For this review, take the finished solid that the model builds, in its own axes (mm). A direction names the side the tool comes from. Give positions to 0.01 mm unless a question says otherwise; leave off trailing zeros. Order: outer loops, then holes, each group sorted by start corner. A loop starts at its lowest first (then second) coordinate and runs counter-clockwise, first axis right, second up. Notation, with made-up numbers: M 83.5,60 L 113.5,60 A16 cw 113.5,81 Z; hole C 63,57.25 d2. An arc over 180 degrees is marked long. Use CSV: the item, a comma, the result in double quotes. Start each with the question number.
(1) Consider section D-D (z = 17). Write out the cut boundary in (x, y), and give its area (3 significant figures).
(2) Consider section B-B (z = 3.5). Write out the cut boundary in (x, y), and give its area (3 significant figures).
(3) Draft analysis for pull direction X (two halves, no side actions). For faces 6 (the face through (30, 2, -37)), 7 (the face through (17.5, 1, 18)), 8 (the face through (-30, 2, 37)), state which applies: pulls with the +X half, pulls with the -X half, needs draft (parallel to the pull), parting line crosses it, or undercut.
(4) Consider section A-A (x = 35). Write out the cut boundary in (y, z), and give its area (3 significant figures).
(5) Wall thickness on L1, parallel to Z at x = 38.5, y = 1.2; L2, parallel to Z at x = -2.5, y = 1.5; L3, parallel to Z at x = 31, y = 3.3: over which ranges is each line inside the solid? List them lowest first. Write a range as from..to.
(6) Consider section C-C (x = 11). Write out the cut boundary in (y, z).
(7) Clearance check with flat-ended pins moving along their axes: P1, Ø1, axis at y = 2, z = 27, coming from the +X side; P2, Ø2, axis at y = 1.5, z = -36, coming from the -X side; P3, Ø0.6, axis at x = 37, y = 2, coming from the -Z side. State where each tip first meets the part, or that it passes through.
(8) Tool access review of faces 1 (the face through (0, 1, 13)), 2 (the face through (37, 2, 13.5)), 3 (the face through (-36, 2, 22.5)), 4 (the face through (-37, 2, 20.5)), 5 (the face through (-35, 2, -22.5)): name each direction out of +Z, -Z, +X, -X, +Y, -Y from which nothing blocks a thin tool from reaching the whole face with its end or side.
```python
from build123d import *

# Parameters (mm, degrees)
SALIENTE_EXTRUIR1_DEPTH = 4
CROQUIS2_W              = 55
CROQUIS2_H              = 101
CORTAR_EXTRUIR1_DEPTH   = 2
CROQUIS4_W              = 7
CROQUIS4_H              = 2
CORTAR_EXTRUIR2_DEPTH   = 9
CROQUIS6_W              = 7
CROQUIS6_H              = 2
CORTAR_EXTRUIR3_DEPTH   = 9
CROQUIS7_W              = 7
CROQUIS7_H              = 2
CORTAR_EXTRUIR4_DEPTH   = 9
CROQUIS8_W              = 7
CROQUIS8_H              = 2
CORTAR_EXTRUIR5_DEPTH   = 9
CROQUIS10_W             = 35
CROQUIS10_H             = 10
CORTAR_EXTRUIR6_DEPTH   = 5


with BuildPart() as part:
    # Croquis1 → Saliente-Extruir1 (new body)
    with BuildSketch(Plane(origin=(0, 0, 0), x_dir=(1, 0, 0), z_dir=(0, 1, 0))):
        Polygon((30, -52.5), (30, -22.5), (41, -22.5), (41, -11.5), (30, -11.5), (30, 11.5), (41, 11.5), (41, 22.5), (30, 22.5), (30, 52.5), (-30, 52.5), (-30, 22.5), (-41, 22.5), (-41, 11.5), (-30, 11.5), (-30, -11.5), (-41, -11.5), (-41, -22.5), (-30, -22.5), (-30, -52.5), align=None)
    extrude(amount=SALIENTE_EXTRUIR1_DEPTH)

    # Croquis2 → Cortar-Extruir1 (cut)
    with BuildSketch(Plane(origin=(0, 4, 0), x_dir=(1, 0, 0), z_dir=(0, 1, 0))):
        Rectangle(CROQUIS2_W, CROQUIS2_H)
    extrude(amount=-CORTAR_EXTRUIR1_DEPTH, mode=Mode.SUBTRACT)

    # Croquis4 → Cortar-Extruir2 (cut)
    with BuildSketch(Plane.ZY.offset(41)):
        with Locations((-17, 2)):
            Rectangle(CROQUIS4_W, CROQUIS4_H)
    extrude(amount=-CORTAR_EXTRUIR2_DEPTH, mode=Mode.SUBTRACT)

    # Croquis6 → Cortar-Extruir3 (cut)
    with BuildSketch(Plane.ZY.offset(41)):
        with Locations((17, 2)):
            Rectangle(CROQUIS6_W, CROQUIS6_H)
    extrude(amount=-CORTAR_EXTRUIR3_DEPTH, mode=Mode.SUBTRACT)

    # Croquis7 → Cortar-Extruir4 (cut)
    with BuildSketch(Plane(origin=(41, 0, 0), x_dir=(0, 0, -1), z_dir=(1, 0, 0))):
        with Locations((-17, 2)):
            Rectangle(CROQUIS7_W, CROQUIS7_H)
    extrude(amount=-CORTAR_EXTRUIR4_DEPTH, mode=Mode.SUBTRACT)

    # Croquis8 → Cortar-Extruir5 (cut)
    with BuildSketch(Plane(origin=(41, 0, 0), x_dir=(0, 0, -1), z_dir=(1, 0, 0))):
        with Locations((17, 2)):
            Rectangle(CROQUIS8_W, CROQUIS8_H)
    extrude(amount=-CORTAR_EXTRUIR5_DEPTH, mode=Mode.SUBTRACT)

    # Croquis10 → Cortar-Extruir6 (cut, through all)
    with BuildSketch(Plane(origin=(0, 0, 0), x_dir=(1, 0, 0), z_dir=(0, 1, 0))):
        with Locations((0, 36)):
            Rectangle(CROQUIS10_W, CROQUIS10_H)
        with Locations((0, 18)):
            Rectangle(CROQUIS10_W, CROQUIS10_H)
        Rectangle(CROQUIS10_W, CROQUIS10_H)
        with Locations((0, -18)):
            Rectangle(CROQUIS10_W, CROQUIS10_H)
        with Locations((0, -36)):
            Rectangle(CROQUIS10_W, CROQUIS10_H)
    extrude(amount=CORTAR_EXTRUIR6_DEPTH, mode=Mode.SUBTRACT)


solid = part.part
```
Check result:
1,outline,"M -41,0 L -17.5,0 L -17.5,2 L -27.5,2 L -27.5,4 L -41,4 L -41,3 L -32,3 L -32,1 L -41,1 Z; M 17.5,0 L 41,0 L 41,1 L 32,1 L 32,3 L 41,3 L 41,4 L 27.5,4 L 27.5,2 L 17.5,2 Z"
1,area,"112 mm^2"
2,outline,"M -30,0 L -17.5,0 L -17.5,2 L -27.5,2 L -27.5,4 L -30,4 Z; M 17.5,0 L 30,0 L 30,4 L 27.5,4 L 27.5,2 L 17.5,2 Z"
2,area,"60.0 mm^2"
3,face 6,"pulls with the +X half"
3,face 7,"undercut"
3,face 8,"pulls with the -X half"
4,outline,"M 0,-22.5 L 4,-22.5 L 4,-11.5 L 0,-11.5 Z; M 0,11.5 L 4,11.5 L 4,22.5 L 0,22.5 Z; hole M 1,-20.5 L 3,-20.5 L 3,-13.5 L 1,-13.5 Z; hole M 1,13.5 L 3,13.5 L 3,20.5 L 1,20.5 Z"
4,area,"60.0 mm^2"
5,L1,"z = -22.5..-20.5, -13.5..-11.5, 11.5..13.5, 20.5..22.5"
5,L2,"z = -52.5..-41, -31..-23, -13..-5, 5..13, 23..31, 41..52.5"
5,L3,"z = -22.5..-11.5, 11.5..22.5"
6,outline,"M 0,-52.5 L 4,-52.5 L 4,-50.5 L 2,-50.5 L 2,-41 L 0,-41 Z; M 0,-31 L 2,-31 L 2,-23 L 0,-23 Z; M 0,-13 L 2,-13 L 2,-5 L 0,-5 Z; M 0,5 L 2,5 L 2,13 L 0,13 Z; M 0,23 L 2,23 L 2,31 L 0,31 Z; M 0,41 L 2,41 L 2,50.5 L 4,50.5 L 4,52.5 L 0,52.5 Z"
7,P1,"stops at x = 30"
7,P2,"stops at x = -30"
7,P3,"stops at z = -22.5"
8,face 1,"+Y, -Y"
8,face 2,"+X"
8,face 3,"+Z, -X, +Y, -Y"
8,face 4,"-X"
8,face 5,"-Z, -X, +Y, -Y"
